Source: CAD feature listing. Evaluate the final solid. Frame: model axes, mm. Face numbers are marked on the shaded views. A direction names the side the tool comes from. Give positions to 0.01 mm unless a question says otherwise; leave off trailing zeros. Loops run counter-clockwise (first coordinate to the right, second up) from the corner with the lowest first, then second, coordinate; pieces in that order, holes last. Notation, with made-up numbers: M 67.5,19 L 80.5,19 A24 cw 80.5,33 Z; hole C 38,50 d2. An arc over 180 degrees is marked long. Put each result on its own line as item: value. Start each with the question number.
```python
from build123d import *

# Parameters (mm, degrees)
F0_R     = 5.5
F0_R_2   = 3.85
F1_DEPTH = 25
F2_START = 11
F2_DEPTH = 14


# Not quite as in the source:
# - a fillet or chamfer that OpenCascade refuses, or shapes differently, is made with other operations: its cross-section is extruded or revolved along the edge and cut away or added


with BuildPart() as f1:
    # F0 (on Top) → F1 (new body)
    with BuildSketch(Plane.XY):
        Circle(F0_R)
        Circle(F0_R_2, mode=Mode.SUBTRACT)
    extrude(amount=F1_DEPTH)

    # F0 (on Top) → F2 (join)
    with BuildSketch(Plane.XY.offset(F2_START)):
        Circle(F0_R_2)
    extrude(amount=F2_DEPTH)

    # F3 (on Front) → F4 (revolve, cut)
    with BuildSketch(Plane.XZ):
        with BuildLine():
            Line((0, 22.2), (0, 31.8))
            ThreePointArc((0, 31.8), (-4.8, 27), (0, 22.2))
        make_face()
    revolve(axis=Axis((0, 0, 27), (0, 0, -1)), mode=Mode.SUBTRACT)

    # F5: fillet of radius 3 on 1 edges, made by hand

    # F5_s1 → F5_t2 (revolve, cut)
    with BuildSketch(Plane.XZ):
        with BuildLine():
            ThreePointArc((5.5, 22.6489525251), (5.2009678393, 23.9546219822), (4.3634848459, 25))
            Line((4.3634848459, 25), (5.5, 25))
            Line((5.5, 25), (5.5, 22.6489525251))
        make_face()
    revolve(axis=Axis((0, 0, 25), (0, 0, 1)), mode=Mode.SUBTRACT)


solid = f1.part
```
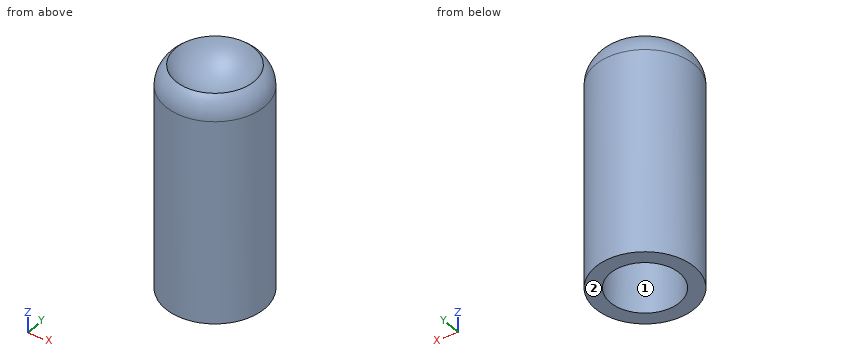
1. Set-up query: the marked faces 1 and 2. Return all of +Z, -Z, +X, -X, +Y, -Y with unobstructed straight access to the full face (end or side cutting, diameter ignored); none if empty.
2. Ray query, line 1 (Y direction, x = 0, z = 2.75); line 2 (Y direction, x = -1.25, z = 6); line 3 (Z direction, x = 3.5, y = 1.5). Return the intervals inside material, ascending.
3. Contact query for flat-ended pins moving along their axis: pin 1 (1 mm diameter, centred on y = -1.5, z = 3.5, fed in from -X); pin 2 (4 mm diameter, centred on x = -3.5, z = 13, fed in from -Y); pin 3 (2.5 mm diameter, centred on x = -1, y = -0.5, fed in from -Z). Output: stop coordinate, or through.
4. Section A-A, the plane z = 9. Output: boundary loops of the cut face in (x, y).
Results found:
1. face 1: -Z
1. face 2: -Z, +X, -X, +Y, -Y
2. line 1: -5.5 to -3.85, 3.85 to 5.5
2. line 2: -5.36 to -3.64, 3.64 to 5.36
2. line 3: 11 to 24.08
3. pin 1: x = -5.41
3. pin 2: y = -5.29
3. pin 3: z = 11
4. outline: C 0,0 d11; hole C 0,0 d7.7
